Build history of the part. All positions in model axes, mm. Face numbers are marked on the shaded views. A direction names the side the tool comes from. Round coordinates to 2 decimals unless told otherwise and drop trailing zeros. Write each loop counter-clockwise with the first axis right and the second up, starting at its lowest first coordinate (ties: lowest second). Pieces come first, ordered by that corner, then holes. Notation, with made-up numbers: (26, 26) -> (67, 26) arc R16 cw to (67, 37) -> close; hole circle Ø10 at (9.5, -15.75). An arc over 180 degrees is marked (long way). Answer in a Markdown table with one row per item.
```python
from build123d import *

# Parameters (mm, degrees)
F0_R     = 13.5636
F0_R_2   = 11
F1_DEPTH = 7


# Not quite as in the source:
# - a feature names something its author has since deleted; it is built from what else it names


with BuildPart() as f1:
    # F0 (on Top) → F1 (new body)
    with BuildSketch(Plane.XY):
        with BuildLine():
            Line((-7.4638039729, 51.7525), (-13.5636, 45.6527039729))
            ThreePointArc((-13.5636, 45.6527039729), (-16.2887093259, 44.7528610649), (-18.9546720538, 43.6905142146))
            ThreePointArc((-18.9546720538, 43.6905142146), (-23.0957546511, 45.8462253684), (-27.5482602123, 44.4423557574))
            Line((-27.5482602123, 44.4423557574), (-38.9834713283, 34.8470743276))
            Line((-38.9834713283, 34.8470743276), (-39.7353128712, 26.2534861691))
            ThreePointArc((-39.7353128712, 26.2534861691), (-41.2444598552, 23.8125), (-42.6038423959, 21.2850472892))
            ThreePointArc((-42.6038423959, 21.2850472892), (-47.1617601278, 20.2745812553), (-49.6701872794, 16.3371393342))
            Line((-49.6701872794, 16.3371393342), (-52.2623391961, 1.6363152952))
            Line((-52.2623391961, 1.6363152952), (-47.3144312411, -5.4300295883))
            ThreePointArc((-47.3144312411, -5.4300295883), (-46.9014692372, -8.2699944614), (-46.318201392, -11.0799298197))
            ThreePointArc((-46.318201392, -11.0799298197), (-49.1602538961, -14.783764754), (-48.5508816958, -19.4124061506))
            Line((-48.5508816958, -19.4124061506), (-41.0870777229, -32.3400938494))
            Line((-41.0870777229, -32.3400938494), (-32.754601392, -34.5727741532))
            ThreePointArc((-32.754601392, -34.5727741532), (-30.6127599113, -36.4828666035), (-28.3597591873, -38.2604846263))
            ThreePointArc((-28.3597591873, -38.2604846263), (-28.156118511, -42.9246229316), (-24.7140789838, -46.0786710526))
            Line((-24.7140789838, -46.0786710526), (-10.6867159511, -51.1842136618))
            Line((-10.6867159511, -51.1842136618), (-2.8685295247, -47.5385334583))
            ThreePointArc((-2.8685295247, -47.5385334583), (0, -47.625), (2.8685295247, -47.5385334583))
            ThreePointArc((2.8685295247, -47.5385334583), (6.0225776457, -50.9805729855), (10.6867159511, -51.1842136618))
            Line((10.6867159511, -51.1842136618), (24.7140789838, -46.0786710526))
            Line((24.7140789838, -46.0786710526), (28.3597591873, -38.2604846263))
            ThreePointArc((28.3597591873, -38.2604846263), (30.6127599113, -36.4828666035), (32.754601392, -34.5727741532))
            ThreePointArc((32.754601392, -34.5727741532), (37.3832427886, -35.1821463535), (41.0870777229, -32.3400938494))
            Line((41.0870777229, -32.3400938494), (48.5508816958, -19.4124061506))
            Line((48.5508816958, -19.4124061506), (46.318201392, -11.0799298197))
            ThreePointArc((46.318201392, -11.0799298197), (46.9014692372, -8.2699944614), (47.3144312411, -5.4300295883))
            ThreePointArc((47.3144312411, -5.4300295883), (51.2518731622, -2.9216024367), (52.2623391961, 1.6363152952))
            Line((52.2623391961, 1.6363152952), (49.6701872794, 16.3371393342))
            Line((49.6701872794, 16.3371393342), (42.6038423959, 21.2850472892))
            ThreePointArc((42.6038423959, 21.2850472892), (41.2444598552, 23.8125), (39.7353128712, 26.2534861691))
            ThreePointArc((39.7353128712, 26.2534861691), (41.1391824821, 30.7059917302), (38.9834713283, 34.8470743276))
            Line((38.9834713283, 34.8470743276), (27.5482602123, 44.4423557574))
            Line((27.5482602123, 44.4423557574), (18.9546720538, 43.6905142146))
            ThreePointArc((18.9546720538, 43.6905142146), (16.2887093259, 44.7528610649), (13.5636, 45.6527039729))
            ThreePointArc((13.5636, 45.6527039729), (11.7770111075, 49.9659111075), (7.4638039729, 51.7525))
            Line((7.4638039729, 51.7525), (-7.4638039729, 51.7525))
        make_face()
        with BuildLine():
            ThreePointArc((26.9782471716, -31.2377944892), (0, -41.275), (-26.9782471716, -31.2377944892))
            Line((-26.9782471716, -31.2377944892), (0, -15.6618962224))
            Line((0, -15.6618962224), (26.9782471716, -31.2377944892))
        make_face(mode=Mode.SUBTRACT)
        Circle(F0_R, mode=Mode.SUBTRACT)
        with BuildLine():
            ThreePointArc((-40.5418471716, -7.7449501556), (-35.7451985412, 20.6375), (-13.5636, 38.9827446448))
            Line((-13.5636, 38.9827446448), (-13.5636, 7.8309481112))
            Line((-13.5636, 7.8309481112), (-40.5418471716, -7.7449501556))
        make_face(mode=Mode.SUBTRACT)
        with BuildLine():
            ThreePointArc((13.5636, 38.9827446448), (35.7451985412, 20.6375), (40.5418471716, -7.7449501556))
            Line((40.5418471716, -7.7449501556), (13.5636, 7.8309481112))
            Line((13.5636, 7.8309481112), (13.5636, 38.9827446448))
        make_face(mode=Mode.SUBTRACT)
        Circle(F0_R)
        Circle(F0_R_2, mode=Mode.SUBTRACT)
    extrude(amount=F1_DEPTH)


solid = f1.part
```
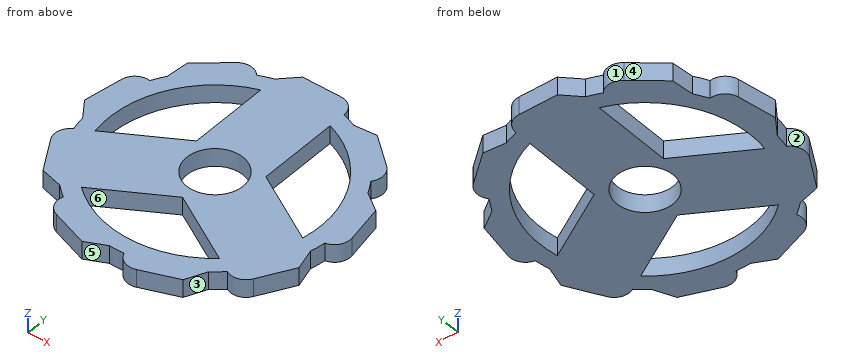
Q1. Saw through at A-A on y = -29.5. Write the cut outline in (x, z).
A:
| item | result |
|---|---|
| outline | (-42.73, 0) -> (-23.97, 0) -> (-23.97, 7) -> (-42.73, 7) -> close; (23.97, 0) -> (42.73, 0) -> (42.73, 7) -> (23.97, 7) -> close |
Q2. Saw through at B-B on z = 1.25. State how many separate pieces and enclosed holes the cut face has, plus the area to 3 significant figures.
A:
| item | result |
|---|---|
| separate pieces | 1 |
| enclosed holes | 4 |
| area | 5,300 mm² |
Q3. Drop flat-ended pins along their axis: P1, Ø1.5, axis at x = 31.5, z = 1, coming from the -Y side; P2, Ø3, axis at x = 30.5, z = 4, coming from the +Y side; P3, Ø13, axis at x = 0, y = 0, coming from the -Z side; P4, Ø2, axis at x = 38, z = 4.5, coming from the +Y side. Give the stop position or say it passes through.
A:
| item | result |
|---|---|
| P1 | y = -36.37 |
| P2 | y = 43.22 |
| P3 | through |
| P4 | y = 36.51 |
Q4. Saw through at C-C on y = 4. Write the cut outline in (x, z).
A:
| item | result |
|---|---|
| outline | (-51.85, 0) -> (-41.08, 0) -> (-41.08, 7) -> (-51.85, 7) -> close; (-20.2, 0) -> (-10.25, 0) -> (-10.25, 7) -> (-20.2, 7) -> close; (10.25, 0) -> (20.2, 0) -> (20.2, 7) -> (10.25, 7) -> close; (41.08, 0) -> (51.85, 0) -> (51.85, 7) -> (41.08, 7) -> close |
Q5. Saw through at D-D on y = 19.5. Write the cut outline in (x, z), plus the area to 3 significant figures.
A:
| item | result |
|---|---|
| outline | (-48.07, 0) -> (-36.38, 0) -> (-36.38, 7) -> (-48.07, 7) -> close; (-13.56, 0) -> (13.56, 0) -> (13.56, 7) -> (-13.56, 7) -> close; (36.38, 0) -> (45.15, 0) -> (45.15, 7) -> (36.38, 7) -> close |
| area | 333 mm² |
Q6. Two-plate mould, pull along Y, no slides. Class the marked faces 1, 2 and 3: released by +Y, released by -Y, zero draft, split by the parting line, or undercut.
A:
| item | result |
|---|---|
| face 1 | released by +Y |
| face 2 | undercut |
| face 3 | released by -Y |
Q7. Wall check: line 1 (Y direction, x = 0, z = 5.75) (1 decimal); line 2 (Y direction, x = 14.5, z = 0.75); line 3 (X direction, y = 1, z = 3.75). Give the ranges that are in metal, low to high. Write a range as [from, to].
A:
| item | result |
|---|---|
| line 1 | [-47.6, -41.3], [-15.7, -11], [11, 51.8] |
| line 2 | [-49.8, -38.64], [-24.03, 7.29], [38.64, 45.36] |
| line 3 | [-51.82, -41.26], [-25.4, -10.95], [10.95, 25.4], [41.26, 52.34] |
Q8. Which spindle directions (+Z, -Z, +X, -X, +Y, -Y) get a long thin tool onto all of the face, cutting with end or side? Do the marked faces 4, 5 and 6. Say none if no direction does.
A:
| item | result |
|---|---|
| face 4 | +Z, -Z, -X, +Y |
| face 5 | +Z, -Z, -Y |
| face 6 | +Z, -Z |
